```python
from build123d import *

# Parameters (mm, degrees)
F1_DEPTH = 12.5
F2_R     = 10
F3_R     = 5
F4_DEPTH = 25.0010001


with BuildPart() as f1:
    # F0 (on Front) → F1 (new body, symmetric)
    with BuildSketch(Plane.XZ):
        with BuildLine():
            ThreePointArc((30.5734569437, 21.7143669149), (0.2987295857, 44.1480604907), (-30.2768086166, 22.1261126273))
            ThreePointArc((-30.2768086166, 22.1261126273), (-0.2537394144, -37.499141541), (30.5734569437, 21.7143669149))
        make_face()
    extrude(amount=F1_DEPTH, both=True)

    # F2
    f2_edges = [f1.edges().sort_by_distance(p)[0] for p in [
        (-30.276809, 0, 22.126113),
        (30.573457, 0, 21.714367),
    ]]
    fillet(f2_edges, radius=F2_R)

    # F3 (on face) → F4 (cut, through all)
    with BuildSketch(Plane.XZ.offset(12.5)):
        Circle(F3_R)
    extrude(amount=-F4_DEPTH, mode=Mode.SUBTRACT)


solid = f1.part
```
For this review, take the finished solid that the model builds, in its own axes (mm). Give positions to 0.01 mm unless a question says otherwise; leave off trailing zeros. Write each loop counter-clockwise with the first axis right and the second up, starting at its lowest first coordinate (ties: lowest second). Pieces come first, ordered by that corner, then holes.
Item 1: The part is to be moulded in two halves that separate along X. For faces 1 (the face through (-1.388, -0.175, -37.474)), 2 (the face through (-0.5, 12.5, -5.2)), 3 (the face through (-1.08, -0.18, -4.88)), say which applies: +X half, -X half, draft (parallel to the pull), parting line (faces both ways), or undercut.
Item 2: Insertion check: P1, Ø5, axis at x = -12, y = 2.5, coming from the +Z side; P2, Ø13, axis at x = 0, z = 0, coming from the +Y side; P3, Ø5, axis at x = 19, y = 8, coming from the +Z side; P4, Ø6, axis at x = -8.5, y = 7.5, coming from the -Z side. Each pin has a flat end and moves straight along its axis. Give the tip position at first contact, or say it passes through.
Item 3: Take a section at A-A (z = 0). Give the boundary of the cut face in (x, y), and give its area (4 significant figures).
Item 4: Wall thickness on probe 1 along Z at (x, y) = (0, 7.5); probe 2 along Z at (x, y) = (-2, -1); probe 3 along X at (y, z) = (-2.75, -4): over which ranges is each line inside the solid? List them lowest first.
Item 5: Take a section at D-D (x = 15.5). Give the boundary of the cut face in (y, z).
Item 6: Take a section at B-B (x = 0). Give the boundary of the cut face in (y, z).
Item 7: Take a section at C-C (z = 10.5). Give the boundary of the cut face in (x, y).
Established:
1. face 1: parting line
1. face 2: draft
1. face 3: undercut
2. P1: stops at z = 42.68
2. P2: stops at y = 12.5
2. P3: stops at z = 39.61
2. P4: stops at z = -37.09
3. outline: (-37.5, -12.5) - (-5, -12.5) - (-5, 12.5) - (-37.5, 12.5) - close; (5, -12.5) - (37.5, -12.5) - (37.5, 12.5) - (5, 12.5) - close
3. area: 1,625 mm2
4. probe 1: z = -37.5 to -5, 5 to 44.15
4. probe 2: z = -37.45 to -4.58, 4.58 to 44.08
4. probe 3: x = -37.29 to -3, 3 to 37.29
5. outline: (-12.5, -34.15) - (12.5, -34.15) - (12.5, 40.18) - (-12.5, 40.18) - close
6. outline: (-12.5, -37.5) - (12.5, -37.5) - (12.5, -5) - (-12.5, -5) - close; (-12.5, 5) - (12.5, 5) - (12.5, 44.15) - (-12.5, 44.15) - close
7. outline: (-36, -12.5) - (36, -12.5) - (36, 12.5) - (-36, 12.5) - close
